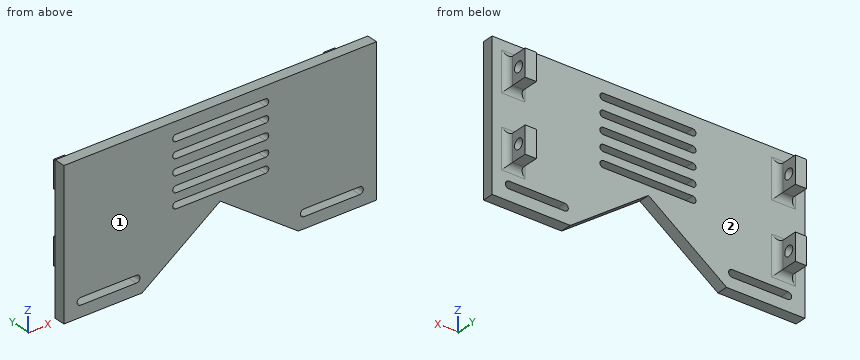
```python
from build123d import *

# Parameters (mm, degrees)
BOSS_EXTRU_1_DEPTH      = 5
ESQUISSE3_W             = 5
ESQUISSE3_H             = 12
BOSS_EXTRU_2_DEPTH      = 10
ESQUISSE4_R             = 2.3
ENL_V_MAT_EXTRU_1_DEPTH = 142.330773303
CONG_1_R                = 2.8


with BuildPart() as part:
    # Esquisse1 → Boss.-Extru.1 (new body)
    with BuildSketch(Plane(origin=(0, 0, 0), x_dir=(1, 0, 0), z_dir=(0, 1, 0))):
        Polygon((70, 45.391491299), (70, 20.391491299), (70, -19.608508701), (-70, -19.608508701), (-70, 20.391491299), (-70, 45.391491299), (-35, 45.391491299), (0, 20.391491299), (35, 45.391491299), align=None)
        with BuildLine():
            ThreePointArc((62.5, 37.191491299), (64.1, 38.791491299), (62.5, 40.391491299))
            Line((62.5, 40.391491299), (37.5, 40.391491299))
            ThreePointArc((37.5, 40.391491299), (35.9, 38.791491299), (37.5, 37.191491299))
            Line((37.5, 37.191491299), (62.5, 37.191491299))
        make_face(mode=Mode.SUBTRACT)
        with BuildLine():
            ThreePointArc((-37.5, 37.194239818), (-35.90137426, 38.792865558), (-37.5, 40.391491299))
            Line((-37.5, 40.391491299), (-62.5, 40.391491299))
            ThreePointArc((-62.5, 40.391491299), (-64.09862574, 38.792865558), (-62.5, 37.194239818))
            Line((-62.5, 37.194239818), (-37.5, 37.194239818))
        make_face(mode=Mode.SUBTRACT)
        with BuildLine():
            ThreePointArc((20.231404284, -14.217017403), (21.731404284, -12.717017403), (20.231404284, -11.217017403))
            Line((20.231404284, -11.217017403), (-19.768595716, -11.217017403))
            ThreePointArc((-19.768595716, -11.217017403), (-21.268595716, -12.717017403), (-19.768595716, -14.217017403))
            Line((-19.768595716, -14.217017403), (20.231404284, -14.217017403))
        make_face(mode=Mode.SUBTRACT)
        with BuildLine():
            ThreePointArc((20.231404284, -7.217017403), (21.731404284, -5.717017403), (20.231404284, -4.217017403))
            Line((20.231404284, -4.217017403), (-19.768595716, -4.217017403))
            ThreePointArc((-19.768595716, -4.217017403), (-21.268595716, -5.717017403), (-19.768595716, -7.217017403))
            Line((-19.768595716, -7.217017403), (20.231404284, -7.217017403))
        make_face(mode=Mode.SUBTRACT)
        with BuildLine():
            ThreePointArc((20.231404284, 13.391491299), (21.731404284, 14.891491299), (20.231404284, 16.391491299))
            Line((20.231404284, 16.391491299), (-19.768595716, 16.391491299))
            ThreePointArc((-19.768595716, 16.391491299), (-21.268595716, 14.891491299), (-19.768595716, 13.391491299))
            Line((-19.768595716, 13.391491299), (20.231404284, 13.391491299))
        make_face(mode=Mode.SUBTRACT)
        with BuildLine():
            ThreePointArc((20.231404284, 6.782982597), (21.731404284, 8.282982597), (20.231404284, 9.782982597))
            Line((20.231404284, 9.782982597), (-19.768595716, 9.782982597))
            ThreePointArc((-19.768595716, 9.782982597), (-21.268595716, 8.282982597), (-19.768595716, 6.782982597))
            Line((-19.768595716, 6.782982597), (20.231404284, 6.782982597))
        make_face(mode=Mode.SUBTRACT)
        with BuildLine():
            ThreePointArc((20.231404284, -0.217017403), (21.731404284, 1.282982597), (20.231404284, 2.782982597))
            Line((20.231404284, 2.782982597), (-19.768595716, 2.782982597))
            ThreePointArc((-19.768595716, 2.782982597), (-21.268595716, 1.282982597), (-19.768595716, -0.217017403))
            Line((-19.768595716, -0.217017403), (20.231404284, -0.217017403))
        make_face(mode=Mode.SUBTRACT)
    extrude(amount=BOSS_EXTRU_1_DEPTH)

    # Esquisse3 → Boss.-Extru.2 (add)
    with BuildSketch(Plane(origin=(0, 5, 0), x_dir=(1, 0, 0), z_dir=(0, 1, 0))):
        with Locations((-60.5, 24.992228824)):
            Rectangle(ESQUISSE3_W, ESQUISSE3_H)
        with Locations((-60.5, -6.608508701)):
            Rectangle(ESQUISSE3_W, ESQUISSE3_H)
        with Locations((60.5, -6.608508701)):
            Rectangle(ESQUISSE3_W, ESQUISSE3_H)
        with Locations((60.5, 24.992228824)):
            Rectangle(ESQUISSE3_W, ESQUISSE3_H)
    extrude(amount=BOSS_EXTRU_2_DEPTH)

    # Esquisse4 → Enlèv. mat.-Extru.1 (cut, through all)
    with BuildSketch(Plane.ZY.offset(63)):
        with Locations((-24.992228824, 11.2)):
            Circle(ESQUISSE4_R)
        with Locations((6.605588836, 11.2)):
            Circle(ESQUISSE4_R)
    extrude(amount=-ENL_V_MAT_EXTRU_1_DEPTH, mode=Mode.SUBTRACT)

    # Congé1
    cong_1_edges = [part.edges().sort_by_distance(p)[0] for p in [
        (-63, 5, -24.992228824),
        (-60.5, 5, -18.992228824),
        (-58, 5, -24.992228824),
        (-60.5, 5, -30.992228824),
        (-63, 5, 6.608508701),
        (-60.5, 5, 12.608508701),
        (-58, 5, 6.608508701),
        (-60.5, 5, 0.608508701),
        (60.5, 5, 0.608508701),
        (58, 5, 6.608508701),
        (60.5, 5, 12.608508701),
        (63, 5, 6.608508701),
        (63, 5, -24.992228824),
        (60.5, 5, -30.992228824),
        (58, 5, -24.992228824),
        (60.5, 5, -18.992228824),
    ]]
    fillet(cong_1_edges, radius=CONG_1_R)


solid = part.part
```
Part model, mm, in its own coordinate system. Face numbers are marked on the shaded views. Coordinates: 2 decimals unless noted, no trailing zeros. Loops run counter-clockwise (first coordinate to the right, second up) from the corner with the lowest first, then second, coordinate; pieces in that order, holes last. Notation, with made-up numbers: (57, 60.25) - (102, 60.25) arc R28 cw to (102, 98.25) - close; hole circle Ø2 at (56.5, 56.5). An arc over 180 degrees is marked (long way). Write item = value, one per line. Start each with the question number.
Item 1: Cut at C-C, the plane x = 16.5. Give the cut face in (y, z), and give its area (3 significant figures).
Item 2: Flat gauge pins, fed straight in: pin 1 Ø7.5 at (y, z) = (11.2, -24.99) entering from -X; pin 2 Ø1 at (x, z) = (37, -34) entering from +Y; pin 3 Ø4 at (x, y) = (-6, 3) entering from -Z. Where does each tip first touch, or does it go through?
Item 3: Cut at A-A, the plane y = 11.2. State how many separate pieces and enclosed holes the cut face has, and give its area (3 significant figures).
Item 4: Mould opens along X. For the marked faces 1 and 2 say: released by +X, released by -X, zero draft, split by the parting line, or undercut.
Item 5: Cut at B-B, the plane x = 47. Give the cut face in (y, z), and give its area (3 significant figures).
Item 6: Wall check: L1, parallel to Z at x = -49.5, y = 4.75; L2, parallel to Z at x = 14.5, y = 1; L3, parallel to X at y = 7.75, z = -20. Give the ranges that are in metal, low to high. Write a range as from..to.
The answers:
q1.outline = (0, -32.18) - (5, -32.18) - (5, -16.39) - (0, -16.39) - close; (0, -13.39) - (5, -13.39) - (5, -9.78) - (0, -9.78) - close; (0, -6.78) - (5, -6.78) - (5, -2.78) - (0, -2.78) - close; (0, 0.22) - (5, 0.22) - (5, 4.22) - (0, 4.22) - close; (0, 7.22) - (5, 7.22) - (5, 11.22) - (0, 11.22) - close; (0, 14.22) - (5, 14.22) - (5, 19.61) - (0, 19.61) - close
q1.area = 184 mm2
q2.pin_1 = -63.02
q2.pin_2 = 5
q2.pin_3 = -26.11
q3.separate_pieces = 8
q3.enclosed_holes = 0
q3.area = 148 mm2
q4.face_1 = zero draft
q4.face_2 = undercut
q5.outline = (0, -45.39) - (5, -45.39) - (5, -40.39) - (0, -40.39) - close; (0, -37.19) - (5, -37.19) - (5, 19.61) - (0, 19.61) - close
q5.area = 309 mm2
q6.L1 = -45.39..-40.39, -37.19..19.61
q6.L2 = -30.75..-16.39, -13.39..-9.78, -6.78..-2.78, 0.22..4.22, 7.22..11.22, 14.22..19.61
q6.L3 = -63..-58, 58..63
